```python
from build123d import *

# Parameters (mm, degrees)
BASE_FLANGE1_DEPTH                              = 3.175
SKETCH8_W                                       = 25.4
SKETCH8_H                                       = 3.175
CUT_EXTRUDE2_DEPTH                              = 251.830023684
SKETCH11_R                                      = 2.753999953
CUT_EXTRUDE4_DEPTH                              = 251.830023684
CSK_FOR_M3_FLAT_HEAD_MACHINE_SCREW1_D           = 3.4
CSK_FOR_M3_FLAT_HEAD_MACHINE_SCREW1_CSINK_D     = 6.3
CSK_FOR_M3_FLAT_HEAD_MACHINE_SCREW1_CSINK_ANGLE = 90


# Sheet-metal steps are written as plain solids
with BuildPart() as part:
    # Sketch1 → Base-Flange1 (new body)
    with BuildSketch(Plane(origin=(0, 0, 0), x_dir=(0, 0, -1), z_dir=(1, 0, 0))):
        with BuildLine():
            Line((0, -103.1875), (0, 103.1875))
            Line((0, 103.1875), (-203.2, 103.1875))
            ThreePointArc((-203.2, 103.1875), (-228.6, 77.7875), (-203.2, 52.3875))
            Line((-203.2, 52.3875), (-50.8, 52.3875))
            Line((-50.8, 52.3875), (-50.8, -77.7875))
            Line((-50.8, -77.7875), (-177.8, -77.7875))
            Line((-177.8, -77.7875), (-177.8, -103.1875))
            Line((-177.8, -103.1875), (-50.8, -103.1875))
            Line((-50.8, -103.1875), (0, -103.1875))
        make_face()
    extrude(amount=-BASE_FLANGE1_DEPTH)

    # Sketch8 → Cut-Extrude2 (cut, through all)
    with BuildSketch(Plane(origin=(0, 0, 0), x_dir=(0, 0, -1), z_dir=(1, 0, 0))):
        with Locations((-38.1, 6.35)):
            Rectangle(SKETCH8_W, SKETCH8_H)
        with Locations((-38.1, -28.575)):
            Rectangle(SKETCH8_W, SKETCH8_H)
    extrude(amount=-CUT_EXTRUDE2_DEPTH, mode=Mode.SUBTRACT)

    # Sketch11 → Cut-Extrude4 (cut, through all)
    with BuildSketch(Plane(origin=(0, 0, 0), x_dir=(0, 0, -1), z_dir=(1, 0, 0))):
        with Locations((-203.2, 77.7875)):
            Circle(SKETCH11_R)
    extrude(amount=-CUT_EXTRUDE4_DEPTH, mode=Mode.SUBTRACT)

    # CSK for M3 Flat Head Machine Screw1 (through all)
    with Locations(Plane(origin=(0, 0, 0), x_dir=(0, 0, -1), z_dir=(1, 0, 0))):
        with Locations((-211.2, 63.931093539), (-219.2, 77.7875), (-211.2, 91.643906461), (-195.2, 91.643906461), (-187.2, 77.7875), (-195.2, 63.931093539)):
            CounterSinkHole(CSK_FOR_M3_FLAT_HEAD_MACHINE_SCREW1_D / 2, CSK_FOR_M3_FLAT_HEAD_MACHINE_SCREW1_CSINK_D / 2, counter_sink_angle=CSK_FOR_M3_FLAT_HEAD_MACHINE_SCREW1_CSINK_ANGLE)


solid = part.part
```
The listing builds one solid part. Answer for the finished solid, in the listing's coordinates (mm). Round coordinates to 2 decimals unless told otherwise and drop trailing zeros. Write each loop counter-clockwise with the first axis right and the second up, starting at its lowest first coordinate (ties: lowest second). Pieces come first, ordered by that corner, then holes. Notation, with made-up numbers: (-13.5, -29.75) -> (41.5, -29.75) arc R17 cw to (41.5, 0.25) -> close; hole circle Ø10 at (27.25, -30). An arc over 180 degrees is marked (long way). Answer as a JSON object with one key per item and string values. Group by question number.
Q1. Section C-C (x = -0.8) is taken. Write down the section's boundary in (y, z).
Q2. Section D-D (y = 1) is taken. Write down the section's boundary in (x, z) (3 decimals), plus the area to 3 significant figures.
Q3. Section A-A (z = 138.5) is taken. Write down the section's boundary in (x, y) (1 decimal).
Q4. Straight lines are drawn through the part: line 1 along Y through (x, z) = (-1.45, 38.5); line 2 along Y through (x, z) = (-0.2, 82); line 3 along Y through (x, z) = (-2.5, 211.2). For each, find the intervals that lie inside material, in ascending order.
Q5. Determine the mould class of faces 1 (the face through (-1.565, 78.346, 228.594)), 2 (the face through (-1.57, 77.91, 205.95)), 3 (the face through (-3.175, 24, 40)) for opening direction Y: pulls with the +Y half, pulls with the -Y half, needs draft (parallel to the pull), parting line crosses it, or undercut.
Q6. Each of these flat-tipped pins is pushed along its axis until it touches: pin 1 Ø1 at (x, y) = (-2.5, -28) entering from +Z; pin 2 Ø1.6 at (x, y) = (-1.5, -43.5) entering from +Z; pin 3 Ø5.5 at (y, z) = (63.93, 211.2) entering from +X. Where does it stop, or does it pass through?
Q7. Section B-B (z = 32) is taken. Write down the section's boundary in (x, y) (1 decimal), plus the area to 3 significant figures.
Check values:
{
 "1": {"outline": "(-103.19, 0) -> (103.19, 0) -> (103.19, 203.2) arc R25.4 ccw to (52.39, 203.2) -> (52.39, 50.8) -> (7.94, 50.8) -> (7.94, 25.4) -> (4.76, 25.4) -> (4.76, 50.8) -> (-26.99, 50.8) -> (-26.99, 25.4) -> (-30.16, 25.4) -> (-30.16, 50.8) -> (-77.79, 50.8) -> (-77.79, 177.8) -> (-103.19, 177.8) -> close; hole circle Ø4.7 at (63.93, 195.2); hole circle Ø4.7 at (63.93, 211.2); hole circle Ø5.51 at (77.79, 203.2); hole circle Ø4.7 at (77.79, 187.2); hole circle Ø4.7 at (77.79, 219.2); hole circle Ø4.7 at (91.64, 195.2); hole circle Ø4.7 at (91.64, 211.2)"},
 "2": {"outline": "(-3.175, 0) -> (0, 0) -> (0, 50.8) -> (-3.175, 50.8) -> close", "area": "161 mm^2"},
 "3": {"outline": "(-3.2, -103.2) -> (0, -103.2) -> (0, -77.8) -> (-3.2, -77.8) -> close; (-3.2, 52.4) -> (0, 52.4) -> (0, 103.2) -> (-3.2, 103.2) -> close"},
 "4": {"line 1": "-103.19 to -30.16, -26.99 to 4.76, 7.94 to 103.19", "line 2": "-103.19 to -77.79, 52.39 to 103.19", "line 3": "53.68 to 62.23, 65.63 to 89.94, 93.34 to 101.89"},
 "5": {"face 1": "parting line crosses it", "face 2": "undercut", "face 3": "needs draft"},
 "6": {"pin 1": "z = 25.4", "pin 2": "z = 50.8", "pin 3": "x = -0.4"},
 "7": {"outline": "(-3.2, -103.2) -> (0, -103.2) -> (0, -30.2) -> (-3.2, -30.2) -> close; (-3.2, -27) -> (0, -27) -> (0, 4.8) -> (-3.2, 4.8) -> close; (-3.2, 7.9) -> (0, 7.9) -> (0, 103.2) -> (-3.2, 103.2) -> close", "area": "635 mm^2"}
}
